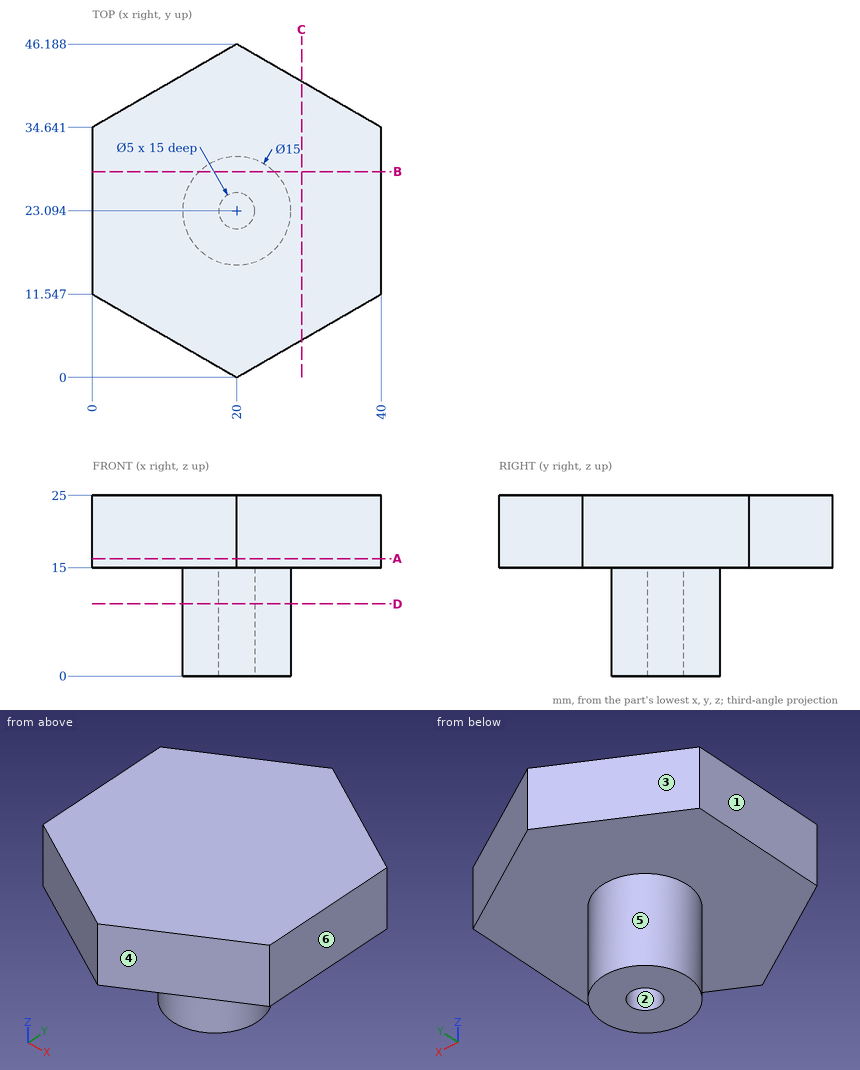
Answer from the drawing. Dimensions are ordinates in mm from the lowest x, y and z of the part. A direction names the side the tool comes from. Coordinates: 2 decimals unless noted, no trailing zeros. Order: outer loops, then holes, each group sorted by start corner. A loop starts at its lowest first (then second) coordinate and runs counter-clockwise, first axis right, second up. Notation, with made-up numbers: (19, -22.75) - (52, -22.75) arc R33 cw to (52, 6.25) - close; hole circle Ø5 at (50, -1). An arc over 180 degrees is marked (long way). Use one line per item in the form item = value.
(1) Section B-B, the plane y = 28.5 is taken. Give the vertices of the cut face in (x, z).
Computed values:
outline = (0, 15) - (14.8, 15) - (14.8, 0) - (25.2, 0) - (25.2, 15) - (40, 15) - (40, 25) - (0, 25) - close
(2) Straight lines are drawn through the part: L1, parallel to Y at x = 20, z = 10; L2, parallel to Z at x = 35, y = 33; L3, parallel to Y at x = 19, z = 11. For each, find the intervals that lie inside material, in ascending order.
Computed values:
L1 = 15.59 to 20.59, 25.59 to 30.59
L2 = 15 to 25
L3 = 15.66 to 20.8, 25.39 to 30.53
(3) Section A-A, the plane z = 16.25 is taken. Give the vertices of the cut face in (x, y), then the cut area to 3 significant figures.
Computed values:
outline = (0, 11.55) - (20, 0) - (40, 11.55) - (40, 34.64) - (20, 46.19) - (0, 34.64) - close
area = 1,390 mm²
(4) Given pin 1 Ø12 at (x, y) = (35.5, 16) entering from -Z; pin 2 Ø10 at (y, z) = (23.5, 7.5) entering from +X; pin 3 Ø1.5 at (x, z) = (35, 15.5) entering from -Y, each flat-ended and moving along its own axis, determine where each tip first touches the part or whether it passes through.
Computed values:
pin_1 = 15
pin_2 = 27.5
pin_3 = 8.23
(5) Section D-D, the plane z = 10 is taken. Give the vertices of the cut face in (x, y), then the cut area to 3 significant figures.
Computed values:
outline = circle Ø15 at (20, 23.09); hole circle Ø5 at (20, 23.09)
area = 157 mm²
(6) For a pull along Y with two mould halves and no side action, classify the marked faces 1, 2, 3 and 4 as pulls with the +Y half, pulls with the -Y half, needs draft (parallel to the pull), parting line crosses it, or undercut.
Computed values:
face_1 = needs draft
face_2 = undercut
face_3 = pulls with the +Y half
face_4 = pulls with the -Y half
(7) Which of the six approach directions +Z, -Z, +X, -X, +Y, -Y give full straight-line access (tool end or side, diameter ignored) to the marked faces 5 and 6?
Computed values:
face_5 = -Z
face_6 = +Z, -Z, +X, +Y, -Y
(8) Section C-C, the plane x = 29 is taken. Give the vertices of the cut face in (y, z), then the cut area to 3 significant figures.
Computed values:
outline = (5.2, 15) - (40.99, 15) - (40.99, 25) - (5.2, 25) - close
area = 358 mm²
